from build123d import *

# Parameters (mm, degrees)
ESQUISSE1_W             = 89.4
ESQUISSE1_H             = 55.2
ESQUISSE1_R             = 1.58
PLAQUE_DEPTH            = 1.6
ESQUISSE2_3_W           = 3.47
ESQUISSE2_3_H           = 51.74
NAPPE_DEPTH             = 2.35
BORDURE_DEPTH           = 2.85
ESQUISSE2_W             = 67.82
ESQUISSE2_H             = 51.74
LCD_DEPTH               = 2.87
SUPPORT_DEPTH           = 1.55
CARTE_SD_DEPTH          = 3
ESQUISSE5_R             = 0.75
ENL_V_MAT_EXTRU_1_DEPTH = 53.735282307


with BuildPart() as part:
    # Esquisse1 → Plaque (new body)
    with BuildSketch(Plane(origin=(0, 0, 0), x_dir=(1, 0, 0), z_dir=(0, 1, 0))):
        Rectangle(ESQUISSE1_W, ESQUISSE1_H)
        with Locations(Location((-41.58, 24.48, 0), (0, 0, 270))):
            Circle(ESQUISSE1_R, mode=Mode.SUBTRACT)
        with Locations(Location((41.58, 24.48, 0), (0, 0, 270))):
            Circle(ESQUISSE1_R, mode=Mode.SUBTRACT)
        with Locations(Location((-41.58, -24.48, 0), (0, 0, 270))):
            Circle(ESQUISSE1_R, mode=Mode.SUBTRACT)
        with Locations(Location((41.58, -24.48, 0), (0, 0, 270))):
            Circle(ESQUISSE1_R, mode=Mode.SUBTRACT)
    extrude(amount=PLAQUE_DEPTH)

    # Esquisse2_3 → Nappe (add)
    with BuildSketch(Plane(origin=(0, 1.6, 0), x_dir=(1, 0, 0), z_dir=(0, 1, 0))):
        with Locations((32.585, 0)):
            Rectangle(ESQUISSE2_3_W, ESQUISSE2_3_H)
    extrude(amount=NAPPE_DEPTH)

    # Esquisse2_5 → Bordure (add)
    with BuildSketch(Plane(origin=(0, 1.6, 0), x_dir=(1, 0, 0), z_dir=(0, 1, 0))):
        Polygon((34.934831333, -20.72), (34.934831333, -25.87), (34.32, -25.87), (30.85, -25.87), (-36.97, -25.87), (-36.97, 25.87), (30.85, 25.87), (34.32, 25.87), (34.934831333, 25.87), (34.934831333, 22.32), (38.77, 22.32), (38.77, 27.47), (-38.77, 27.47), (-38.77, -27.47), (38.77, -27.47), (38.77, -20.72), align=None)
    extrude(amount=BORDURE_DEPTH)

    # Esquisse2 → LCD (add)
    with BuildSketch(Plane(origin=(0, 1.6, 0), x_dir=(1, 0, 0), z_dir=(0, 1, 0))):
        with Locations((-3.06, 0)):
            Rectangle(ESQUISSE2_W, ESQUISSE2_H)
    extrude(amount=LCD_DEPTH)

    # Esquisse2_8 → Support (add)
    with BuildSketch(Plane(origin=(0, 1.6, 0), x_dir=(1, 0, 0), z_dir=(0, 1, 0))):
        Polygon((34.32, -25.87), (34.934831333, -25.87), (34.934831333, -20.72), (38.77, -20.72), (38.77, 22.32), (34.934831333, 22.32), (34.934831333, 25.87), (34.32, 25.87), align=None)
    extrude(amount=SUPPORT_DEPTH)

    # Esquisse4 → Carte SD (add)
    with BuildSketch(Plane.XZ):
        Polygon((-15.04, 26.3), (11.5, 26.3), (11.5, 9.7), (-12.95, 9.7), (-12.95, 15.282856636), (-15.04, 17.558065393), align=None)
    extrude(amount=CARTE_SD_DEPTH)

    # Esquisse5 → Enl_v. mat.-Extru.1 (cut, through all)
    with BuildSketch(Plane(origin=(0, 1.6, 0), x_dir=(1, 0, 0), z_dir=(0, 1, 0))):
        with Locations(Location((42.724707786, 16.6, 0), (0, 0, 270))):
            Circle(ESQUISSE5_R)
        with Locations(Location((42.724707786, 14.05, 0), (0, 0, 270))):
            Circle(ESQUISSE5_R)
        with Locations(Location((42.724707786, 11.5, 0), (0, 0, 270))):
            Circle(ESQUISSE5_R)
        with Locations(Location((42.724707786, 8.95, 0), (0, 0, 270))):
            Circle(ESQUISSE5_R)
        with Locations(Location((42.724707786, 6.4, 0), (0, 0, 270))):
            Circle(ESQUISSE5_R)
        with Locations(Location((42.724707786, 3.85, 0), (0, 0, 270))):
            Circle(ESQUISSE5_R)
        with Locations(Location((42.724707786, 1.3, 0), (0, 0, 270))):
            Circle(ESQUISSE5_R)
        with Locations(Location((42.724707786, -1.25, 0), (0, 0, 270))):
            Circle(ESQUISSE5_R)
        with Locations(Location((42.724707786, -3.8, 0), (0, 0, 270))):
            Circle(ESQUISSE5_R)
        with Locations(Location((42.724707786, -6.35, 0), (0, 0, 270))):
            Circle(ESQUISSE5_R)
        with Locations(Location((42.724707786, -8.9, 0), (0, 0, 270))):
            Circle(ESQUISSE5_R)
        with Locations(Location((42.724707786, -11.45, 0), (0, 0, 270))):
            Circle(ESQUISSE5_R)
        with Locations(Location((42.724707786, -14, 0), (0, 0, 270))):
            Circle(ESQUISSE5_R)
        with Locations(Location((42.724707786, -16.55, 0), (0, 0, 270))):
            Circle(ESQUISSE5_R)
    extrude(amount=-ENL_V_MAT_EXTRU_1_DEPTH, mode=Mode.SUBTRACT)


solid = part.part
The listing builds one solid part. Answer for the finished solid, in the listing's coordinates (mm). A direction names the side the tool comes from. Give positions to 0.01 mm unless a question says otherwise; leave off trailing zeros. Write each loop counter-clockwise with the first axis right and the second up, starting at its lowest first coordinate (ties: lowest second). Pieces come first, ordered by that corner, then holes.
1) A tool of negligible diameter and unlimited length cuts with its end or side. For faces 1 (the face through (11.5, -1, 18)), 2 (the face through (-2, -1, 26.3)), 3 (the face through (33, 3.95, 0)), 4 (the face through (1, 3, -27.47)), from which of +Z, -Z, +X, -X, +Y, -Y can it reach the whole face along a straight path? Write none if from no direction.
2) Section A-A (x = -41.58) is taken. Write down the section's boundary in (y, z).
3) Section B-B (z = 24.48) is taken. Count the separate pieces of the cut face and the enclosed holes in it, and give its area (3 significant figures).
4) Find the intervals of material crossed by L1, parallel to X at y = 0.5, z = -24.48; L2, parallel to X at y = 1.15, z = 14; L3, parallel to Y at x = -33, z = -6, in increasing order.
5) For a pull along Z with two mould halves and no side action, classify faces 5 (the face through (-38.77, 3, 0)), 6 (the face through (-1, 3, 27.47)), 7 (the face through (-1, 1, -27.6)), 8 (the face through (-40.013, 0.789, 24.274)) as pulls with the +Z half, pulls with the -Z half, needs draft (parallel to the pull), parting line crosses it, or undercut.
6) Given P1, Ø0.9, axis at x = 42.72, z = 11.45, coming from the -Y side; P2, Ø1.7, axis at x = 42.72, z = 3.8, coming from the -Y side; P3, Ø3.5, axis at x = -41.58, z = -24.48, coming from the +Y side; P4, Ø1.4, axis at y = 3.5, z = 4.5, coming from the +X side, each flat-ended and moving along its own axis, determine where each tip first touches the part or whether it passes through.
Response:
1. face 1: +Z, -Z, +X, -Y
1. face 2: +Z, +X, -X, -Y
1. face 3: +Y
1. face 4: -Z, +X, -X, +Y
2. outline: (0, -27.6) - (1.6, -27.6) - (1.6, -26.06) - (0, -26.06) - close; (0, -22.9) - (1.6, -22.9) - (1.6, 22.9) - (0, 22.9) - close; (0, 26.06) - (1.6, 26.06) - (1.6, 27.6) - (0, 27.6) - close
3. separate pieces: 3
3. enclosed holes: 0
3. area: 432 mm2
4. L1: x = -44.7 to -43.16, -40 to 40, 43.16 to 44.7
4. L2: x = -44.7 to 41.97, 43.47 to 44.7
4. L3: y = 0 to 4.47
5. face 5: needs draft
5. face 6: pulls with the +Z half
5. face 7: pulls with the -Z half
5. face 8: undercut
6. P1: passes through
6. P2: stops at y = 0
6. P3: stops at y = 1.6
6. P4: stops at x = 38.77
